```python
from build123d import *

# Parameters (mm, degrees)
SKETCH1_W                = 120
SKETCH1_H                = 80
BOSS_EXTRUDE1_DEPTH      = 100
SKETCH2_W                = 40
SKETCH2_H                = 20
CUT_EXTRUDE1_DEPTH       = 100
CUT_EXTRUDE2_DEPTH       = 100
SKETCH4_W                = 20
SKETCH4_H                = 50
CUT_EXTRUDE3_DEPTH       = 100
SKETCH5_W                = 60
SKETCH5_H                = 30
CUT_EXTRUDE4_DEPTH       = 100
CUT_EXTRUDE5_DEPTH       = 100
SKETCH7_W                = 30
SKETCH7_H                = 20
CUT_EXTRUDE6_DEPTH       = 30
CUT_EXTRUDE7_DEPTH       = 110
CUT_EXTRUDE8_DEPTH       = 110
CUT_EXTRUDE9_DEPTH       = 110
CUT_EXTRUDE11_DEPTH      = 110
CUT_EXTRUDE12_DEPTH      = 110
CUT_EXTRUDE13_DEPTH      = 110
BOSS_EXTRUDE4_DEPTH      = 50
BOSS_EXTRUDE6_DEPTH      = 40
BOSS_EXTRUDE7_DEPTH      = 40
CUT_EXTRUDE18_DEPTH      = 84
CUT_EXTRUDE18_DEPTH_BACK = 20
CUT_EXTRUDE19_DEPTH      = 20
SKETCH34_W               = 40
SKETCH34_H               = 50
BOSS_EXTRUDE8_DEPTH      = 30
SKETCH35_W               = 20
SKETCH35_H               = 14.142135624
CUT_EXTRUDE20_DEPTH      = 30
SKETCH36_W               = 20
SKETCH36_H               = 30
BOSS_EXTRUDE9_DEPTH      = 30
BOSS_EXTRUDE10_DEPTH     = 30
BOSS_EXTRUDE11_DEPTH     = 30
BOSS_EXTRUDE12_DEPTH     = 30
BOSS_EXTRUDE13_DEPTH     = 30
SKETCH41_W               = 40
SKETCH41_H               = 20
CUT_EXTRUDE21_DEPTH      = 172


with BuildPart() as part:
    # Sketch1 → Boss-Extrude1 (new body)
    with BuildSketch(Plane.XY):
        with Locations((60, 40)):
            Rectangle(SKETCH1_W, SKETCH1_H)
    extrude(amount=-BOSS_EXTRUDE1_DEPTH)

    # Sketch2 → Cut-Extrude1 (cut)
    with BuildSketch(Plane.XY):
        with Locations((60, 10)):
            Rectangle(SKETCH2_W, SKETCH2_H)
    extrude(amount=-CUT_EXTRUDE1_DEPTH, mode=Mode.SUBTRACT)

    # Sketch3 → Cut-Extrude2 (cut)
    with BuildSketch(Plane.XY):
        Polygon((0, 50), (10, 60), (10, 80), (0, 80), align=None)
    extrude(amount=-CUT_EXTRUDE2_DEPTH, mode=Mode.SUBTRACT)

    # Sketch4 → Cut-Extrude3 (cut)
    with BuildSketch(Plane(origin=(0, 0, 0), x_dir=(-1, 0, 0), z_dir=(0, -1, 0))):
        with Locations((-10, 25)):
            Rectangle(SKETCH4_W, SKETCH4_H)
    extrude(amount=-CUT_EXTRUDE3_DEPTH, mode=Mode.SUBTRACT)

    # Sketch5 → Cut-Extrude4 (cut)
    with BuildSketch(Plane(origin=(0, 0, 0), x_dir=(-1, 0, 0), z_dir=(0, -1, 0))):
        with Locations((-50, 15)):
            Rectangle(SKETCH5_W, SKETCH5_H)
    extrude(amount=-CUT_EXTRUDE4_DEPTH, mode=Mode.SUBTRACT)

    # Sketch6 → Cut-Extrude5 (cut)
    with BuildSketch(Plane.XZ):
        Polygon((80, -30), (100, -10), (100, 0), (80, 0), align=None)
    extrude(amount=-CUT_EXTRUDE5_DEPTH, mode=Mode.SUBTRACT)

    # Sketch7 → Cut-Extrude6 (cut)
    with BuildSketch(Plane(origin=(0, 80, 0), x_dir=(1, 0, 0), z_dir=(0, 1, 0))):
        with Locations((105, 10)):
            Rectangle(SKETCH7_W, SKETCH7_H)
    extrude(amount=-CUT_EXTRUDE6_DEPTH, mode=Mode.SUBTRACT)

    # Sketch9 → Cut-Extrude7 (cut)
    with BuildSketch(Plane.XY.offset(-90)):
        Polygon((10, 80), (10, 60), (30, 80), align=None)
    extrude(amount=CUT_EXTRUDE7_DEPTH, mode=Mode.SUBTRACT)

    # Sketch15 → Cut-Extrude8 (cut)
    with BuildSketch(Plane(origin=(6.578947368, -3.947368421, -2.631578947), x_dir=(0.278207442, -0.166924465, 0.945905303), z_dir=(-0.811107106, 0.486664263, 0.324442842))):
        Polygon((-71.221105162, 84.03430672), (-71.221105162, 25.724787771), (-50.077339567, 14.291548762), (-50.077339567, 53.164561394), align=None)
    extrude(amount=CUT_EXTRUDE8_DEPTH, mode=Mode.SUBTRACT)

    # Sketch18 → Cut-Extrude9 (cut)
    with BuildSketch(Plane(origin=(12.371134021, -10.309278351, -12.371134021), x_dir=(-0.468006318, 0.390005265, -0.793010706), z_dir=(0.609207699, -0.507673083, -0.609207699))):
        Polygon((72.670981065, 80.663234358), (22.230300111, 106.270610344), (22.230300111, 28.168113585), align=None)
    extrude(amount=-CUT_EXTRUDE9_DEPTH, mode=Mode.SUBTRACT)

    # Sketch19 → Cut-Extrude11 (cut)
    with BuildSketch(Plane(origin=(11.193675889, -9.328063241, -7.928853755), x_dir=(0.367189278, -0.305991065, 0.878374352), z_dir=(-0.674785869, 0.562321557, 0.477973324))):
        Polygon((-25.127266295, 106.270610344), (-70.665936585, 106.270610344), (-70.665936585, 23.046638388), (-25.127266295, 28.168113585), align=None)
    extrude(amount=CUT_EXTRUDE11_DEPTH, mode=Mode.SUBTRACT)

    # Sketch20 → Cut-Extrude12 (cut)
    with BuildSketch(Plane(origin=(18.330133634, 24.566158479, -3.023527197), x_dir=(0.803624389, -0.590679852, 0.072699059), z_dir=(0.595136826, 0.797606055, -0.098166899))):
        Polygon((-14.663450209, 46.256870976), (-22.809329684, 65.811114724), (-10.365705355, 46.571670512), align=None)
    extrude(amount=-CUT_EXTRUDE12_DEPTH, mode=Mode.SUBTRACT)

    # Sketch23 → Cut-Extrude13 (cut)
    with BuildSketch(Plane.XY.offset(-70)):
        Polygon((0, 30), (0, 80), (41.666666667, 80), align=None)
    extrude(amount=CUT_EXTRUDE13_DEPTH, mode=Mode.SUBTRACT)

    # Sketch27 → Boss-Extrude4 (add)
    with BuildSketch(Plane.XY.offset(-30)):
        Polygon((20, 20), (70, 80), (20, 30), align=None)
    extrude(amount=-BOSS_EXTRUDE4_DEPTH)

    # Sketch28 → Boss-Extrude6 (add)
    with BuildSketch(Plane(origin=(6.666666667, -6.666666667, -6.666666667), x_dir=(0.816496581, 0.40824829, 0.40824829), z_dir=(-0.577350269, 0.577350269, 0.577350269))):
        Polygon((28.577380332, 106.066017178), (77.567175188, 77.781745931), (16.329931619, 42.426406871), (-8.164965809, 84.852813742), align=None)
    extrude(amount=-BOSS_EXTRUDE6_DEPTH)

    # Sketch29 → Boss-Extrude7 (add)
    with BuildSketch(Plane(origin=(0, 80, 0), x_dir=(1, 0, 0), z_dir=(0, 1, 0))):
        Polygon((30, 70), (41.666666667, 70), (70, 30), align=None)
    extrude(amount=-BOSS_EXTRUDE7_DEPTH)

    # Sketch30 → Cut-Extrude18 (cut, two sides)
    with BuildSketch(Plane.XY.offset(-50)) as cut_extrude18_sk:
        Polygon((0, 0), (0, 30), (20, 50), (20, 0), align=None)
    extrude(amount=CUT_EXTRUDE18_DEPTH, mode=Mode.SUBTRACT)
    extrude(cut_extrude18_sk.sketch, amount=-CUT_EXTRUDE18_DEPTH_BACK, mode=Mode.SUBTRACT)

    # Sketch33 → Cut-Extrude19 (cut)
    with BuildSketch(Plane(origin=(11.193675889, -9.328063241, -7.928853755), x_dir=(0.367189278, -0.305991065, 0.878374352), z_dir=(-0.674785869, 0.562321557, 0.477973324))):
        Polygon((-70.665936585, 37.247092344), (-67.987191274, 37.130695181), (-70.665936585, 23.046638388), align=None)
    extrude(amount=-CUT_EXTRUDE19_DEPTH, mode=Mode.SUBTRACT)

    # Sketch34 → Boss-Extrude8 (add)
    with BuildSketch(Plane(origin=(0, 0, -100), x_dir=(-1, 0, 0), z_dir=(0, 0, -1))):
        with Locations((-20, 25)):
            Rectangle(SKETCH34_W, SKETCH34_H)
    extrude(amount=-BOSS_EXTRUDE8_DEPTH)

    # Sketch35 → Cut-Extrude20 (cut)
    with BuildSketch(Plane(origin=(-15, 15, 0), x_dir=(0, 0, -1), z_dir=(0.707106781, -0.707106781, 0))):
        with Locations((60, 42.426406871)):
            Rectangle(SKETCH35_W, SKETCH35_H)
    extrude(amount=-CUT_EXTRUDE20_DEPTH, mode=Mode.SUBTRACT)

    # Sketch36 → Boss-Extrude9 (add)
    with BuildSketch(Plane.ZY):
        with Locations((-60, 15)):
            Rectangle(SKETCH36_W, SKETCH36_H)
    extrude(amount=-BOSS_EXTRUDE9_DEPTH)

    # Sketch37 → Boss-Extrude10 (add)
    with BuildSketch(Plane.XY.offset(-50)):
        Polygon((0, 30), (20, 50), (20, 30), align=None)
    extrude(amount=-BOSS_EXTRUDE10_DEPTH)

    # Sketch38 → Boss-Extrude11 (add)
    with BuildSketch(Plane(origin=(6.666666667, -6.666666667, -6.666666667), x_dir=(0.816496581, 0.40824829, 0.40824829), z_dir=(-0.577350269, 0.577350269, 0.577350269))):
        Polygon((4.082482905, 91.923881554), (-8.164965809, 56.568542495), (16.329931619, 70.710678119), align=None)
    extrude(amount=-BOSS_EXTRUDE11_DEPTH)

    # Sketch39 → Boss-Extrude12 (add)
    with BuildSketch(Plane(origin=(6.666666667, -6.666666667, -6.666666667), x_dir=(0.816496581, 0.40824829, 0.40824829), z_dir=(-0.577350269, 0.577350269, 0.577350269))):
        Polygon((-8.164965809, 84.852813742), (4.082482905, 91.923881554), (-8.164965809, 56.568542495), align=None)
    extrude(amount=-BOSS_EXTRUDE12_DEPTH)

    # Sketch40 → Boss-Extrude13 (add)
    with BuildSketch(Plane.ZY):
        Polygon((-70, 30), (-70, 50), (-50, 30), align=None)
    extrude(amount=-BOSS_EXTRUDE13_DEPTH)

    # Sketch41 → Cut-Extrude21 (cut)
    with BuildSketch(Plane.XY.offset(-30)):
        with Locations((60, 10)):
            Rectangle(SKETCH41_W, SKETCH41_H)
    extrude(amount=-CUT_EXTRUDE21_DEPTH, mode=Mode.SUBTRACT)


solid = part.part
```
Source: CAD feature listing. Evaluate the final solid. Frame: model axes, mm. A direction names the side the tool comes from. Give positions to 0.01 mm unless a question says otherwise; leave off trailing zeros. Order: outer loops, then holes, each group sorted by start corner. A loop starts at its lowest first (then second) coordinate and runs counter-clockwise, first axis right, second up.
(1) Section query A-A (y = 47.5). Return the cut outline in (x, z).
(2) Section query C-C (z = -37). Return the cut outline in (x, y).
(3) Pull-direction query (X, two-part tool) for faces 4 (the face through (60, 20, -65)), 5 (the face through (0, 25, -75)), 6 (the face through (110, 25, 0)); classes: +X half, -X half, draft (parallel to the pull), parting line (faces both ways), or undercut.
(4) Section query D-D (y = 68). Return the cut outline in (x, z), plus the area to 3 significant figures.
(5) Access query for faces 1 (the face through (100, 25, -5)), 2 (the face through (10, 70, -95)), 3 (the face through (18, 72, -90)). Directions: +Z, -Z, +X, -X, +Y, -Y. A direction counts if a zero-diameter tool reaches every point of the face in a straight line with its end or side. Return the directions, or none.
(6) Contact query for flat-ended pins moving along their axis: P1, Ø22, axis at x = 7.5, y = 28, coming from the +Z side; P2, Ø6, axis at x = 106, y = 66, coming from the +Z side; P3, Ø1.5, axis at x = 34, y = 67.5, coming from the +Z side. Output: stop coordinate, or through.
(7) Material intervals for line 1 along X through (y, z) = (5.5, -74.5); line 2 along X through (y, z) = (29.5, -20); line 3 along Z through (x, y) = (111.5, 74), sorted ascending.
(8) Section query B-B (x = 105). Return the cut outline in (y, z), plus the area to 3 significant figures.
Outcome:
1. outline: (0, -100) - (120, -100) - (120, 0) - (100, 0) - (100, -10) - (80, -30) - (37.5, -30) - (20, -47.5) - (20, -50) - (17.5, -50) - (0, -67.5) - close
2. outline: (20, 0) - (40, 0) - (40, 20) - (80, 20) - (80, 0) - (120, 0) - (120, 80) - (63, 80) - (20, 37) - close
3. face 4: undercut
3. face 5: -X half
3. face 6: draft
4. outline: (10, -100) - (120, -100) - (120, -20) - (90, -20) - (80, -30) - (58, -30) - (18, -70) - (18, -90) - (10, -90) - close
4. area: 6,770 mm2
5. face 1: +Z, -X, +Y, -Y
5. face 2: +Z, -Z, -X, +Y
5. face 3: +Z, -X, +Y
6. P1: stops at z = -50
6. P2: stops at z = -20
6. P3: stops at z = -52.44
7. line 1: x = 0 to 40, 80 to 120
7. line 2: x = 90 to 120
7. line 3: z = -100 to -20
8. outline: (0, -100) - (80, -100) - (80, -20) - (50, -20) - (50, 0) - (0, 0) - close
8. area: 7,400 mm2
